Design review of the part built by this model. Coordinates are the model's own, in mm. A direction names the side the tool comes from. Coordinates: 2 decimals unless noted, no trailing zeros. Write each loop counter-clockwise with the first axis right and the second up, starting at its lowest first coordinate (ties: lowest second). Pieces come first, ordered by that corner, then holes. Notation, with made-up numbers: (-7.5, 34) - (15.5, 34) arc R27 ccw to (15.5, 69) - close; hole circle Ø1 at (64.25, 55.25). An arc over 180 degrees is marked (long way). Answer as a JSON object with one key per item and string values.
```python
from build123d import *

# Parameters (mm, degrees)
BOSS_EXTRUDE1_DEPTH   = 41
SKETCH2_R             = 2.75
SKETCH2_R_2           = 5.237100589
SKETCH2_R_3           = 5.771252778
SKETCH2_R_4           = 5.5
CUT_EXTRUDE10_DEPTH   = 13
SKETCH11_R            = 5
CUT_EXTRUDE11_DEPTH   = 5.7
M5_TAPPED_HOLE1_D     = 4.2
M5_TAPPED_HOLE1_DEPTH = 12
M5_TAPPED_HOLE1_TIP   = 1.2618073


with BuildPart() as part:
    # Sketch1 → Boss-Extrude1 (new body)
    with BuildSketch(Plane(origin=(0, 0, 0), x_dir=(1, 0, 0), z_dir=(0, 1, 0))):
        Polygon((-6, 25), (-5, 25), (-5, -25), (-6, -25), (-6, -35), (6, -35), (6, 35), (-6, 35), align=None)
    extrude(amount=BOSS_EXTRUDE1_DEPTH)

    # Sketch2 → Cut-Extrude10 (cut, through all)
    with BuildSketch(Plane(origin=(6, 0, 0), x_dir=(0, 0, -1), z_dir=(1, 0, 0))):
        with Locations((29, 28)):
            Circle(SKETCH2_R)
        with Locations((-17.5, 20.5)):
            Circle(SKETCH2_R_2)
        with Locations((0, 20.5)):
            Circle(SKETCH2_R_3)
        with Locations((17.5, 20.5)):
            Circle(SKETCH2_R_4)
        with Locations((-29, 13)):
            Circle(SKETCH2_R)
    extrude(amount=-CUT_EXTRUDE10_DEPTH, mode=Mode.SUBTRACT)

    # Sketch11 → Cut-Extrude11 (cut)
    with BuildSketch(Plane(origin=(6, 0, 0), x_dir=(0, 0, -1), z_dir=(1, 0, 0))):
        with Locations((29, 28)):
            Circle(SKETCH11_R)
        with Locations((-29, 13)):
            Circle(SKETCH11_R)
    extrude(amount=-CUT_EXTRUDE11_DEPTH, mode=Mode.SUBTRACT)

    # M5 Tapped Hole1
    with Locations(Plane(origin=(0, 41, 0), x_dir=(1, 0, 0), z_dir=(0, 1, 0))):
        with Locations((0.5, -6.5)):
            Hole(M5_TAPPED_HOLE1_D / 2, depth=M5_TAPPED_HOLE1_DEPTH)
            with Locations((0, 0, -(M5_TAPPED_HOLE1_DEPTH + M5_TAPPED_HOLE1_TIP / 2))):  # 118° drill point
                Cone(0, M5_TAPPED_HOLE1_D / 2, M5_TAPPED_HOLE1_TIP, mode=Mode.SUBTRACT)


solid = part.part
```
(1) For pin 1 (12.5 mm diameter, centred on y = 20.5, z = -17.5, fed in from -X); pin 2 (4 mm diameter, centred on x = 0.5, z = 6.5, fed in from +Y), all flat-tipped, find the tip position at first contact; note any pin that passes through.
Solved:
{"pin 1": "stops at x = -5", "pin 2": "stops at y = 28.94"}
(2) Take a section at D-D, the plane x = -4. Write out the cut boundary in (y, z).
Solved:
{"outline": "(0, -35) - (41, -35) - (41, 35) - (0, 35) - close; hole circle Ø5.5 at (13, 29); hole circle Ø11.54 at (20.5, 0); hole circle Ø11 at (20.5, -17.5); hole circle Ø10.47 at (20.5, 17.5); hole circle Ø5.5 at (28, -29)"}
(3) To check wall thickness, follow line 1 (Y direction, x = -4, z = 29); line 2 (Y direction, x = 0.75, z = -17.5); line 3 (Z direction, x = -2.25, y = 19). State the ranges of each line that lie inside material, in increasing order. Write a range as from..to.
Solved:
{"line 1": "y = 0..10.25, 15.75..41", "line 2": "y = 0..15, 26..41", "line 3": "z = -35..-22.79, -12.21..-5.57, 5.57..12.48, 22.52..35"}
(4) Take a section at B-B, the plane z = -29. Write out the cut boundary in (x, y), and give its area (3 significant figures).
Solved:
{"outline": "(-6, 0) - (6, 0) - (6, 23) - (0.3, 23) - (0.3, 25.25) - (-6, 25.25) - close; (-6, 30.75) - (0.3, 30.75) - (0.3, 33) - (6, 33) - (6, 41) - (-6, 41) - close", "area": "400 mm^2"}
(5) The part is to be moulded in two halves that separate along X. For faces 1 (the face through (0.58, 24.22, -13.45)), 2 (the face through (-6, 20, 30)), 3 (the face through (0.3, 10.8, 26.8)), 4 (the face through (0.773, 34.916, 4.418)), say which applies: pulls with the +X half, pulls with the -X half, needs draft (parallel to the pull), parting line crosses it, or undercut.
Solved:
{"face 1": "needs draft", "face 2": "pulls with the -X half", "face 3": "pulls with the +X half", "face 4": "undercut"}
(6) Take a section at A-A, the plane y = 13. Write out the cut boundary in (x, z), and give its area (3 significant figures).
Solved:
{"outline": "(-6, -35) - (6, -35) - (6, 24) - (0.3, 24) - (0.3, 26.25) - (-6, 26.25) - (-6, 25) - (-5, 25) - (-5, -25) - (-6, -25) - close; (-6, 31.75) - (0.3, 31.75) - (0.3, 34) - (6, 34) - (6, 35) - (-6, 35) - close", "area": "698 mm^2"}
(7) Take a section at C-C, the plane y = 20.5. Write out the cut boundary in (x, z).
Solved:
{"outline": "(-6, -35) - (6, -35) - (6, -23) - (-5, -23) - (-5, -25) - (-6, -25) - close; (-6, 25) - (-5, 25) - (-5, 22.74) - (6, 22.74) - (6, 35) - (-6, 35) - close; (-5, -12) - (6, -12) - (6, -5.77) - (-5, -5.77) - close; (-5, 5.77) - (6, 5.77) - (6, 12.26) - (-5, 12.26) - close"}
(8) Tool access review of faces 5 (the face through (3, 25, -25)), 6 (the face through (-5, 20, -6)), 7 (the face through (0, 41, 0)): name each direction out of +Z, -Z, +X, -X, +Y, -Y from which nothing blocks a thin tool from reaching the whole face with its end or side.
Solved:
{"face 5": "+X", "face 6": "-X, +Y, -Y", "face 7": "+Z, -Z, +X, -X, +Y"}
